Design review of the part built by this model. Coordinates are the model's own, in mm. Face numbers are marked on the shaded views. A direction names the side the tool comes from. Coordinates: 2 decimals unless noted, no trailing zeros. Loops run counter-clockwise (first coordinate to the right, second up) from the corner with the lowest first, then second, coordinate; pieces in that order, holes last.
from build123d import *

# Parameters (mm, degrees)
F_0075_CYLINDER_SKETCH_R    = 3.25
F_0075_CYLINDER_DEPTH       = 2.5
F_0076_FILLET_R             = 0.625
F_0077_EXTRUDE_DEPTH        = 1.385
F_0077_EXTRUDE_ROTATE_ANGLE = 120
F_0080_CYLINDER_SKETCH_R    = 1.2
F_0080_CYLINDER_DEPTH       = 17.7
F_0081_CONE_ROTATE_ANGLE    = 90


with BuildPart() as part:
    # 0075_cylinder_Sketch → 0075_cylinder (new body)
    with BuildSketch(Plane.XY):
        Circle(F_0075_CYLINDER_SKETCH_R)
    extrude(amount=F_0075_CYLINDER_DEPTH)

    # 0076_fillet
    f_0076_fillet_edges = [part.edges().sort_by_distance(p)[0] for p in [
        (-3.25, 0, 2.5),
    ]]
    fillet(f_0076_fillet_edges, radius=F_0076_FILLET_R)


with BuildPart() as body_2:
    # 0077_extrude_Sketch → 0077_extrude (new body)
    with BuildSketch(Plane.XY):
        Polygon((0, 0), (1.154700538, 0), (1.732050808, 1), (1.154700538, 2), (0, 2), (-0.577350269, 1), align=None)
    extrude(amount=F_0077_EXTRUDE_DEPTH)


with BuildPart() as body_2_1:
    # 0077_extrude_Rotate: read off the stored shape, not the designer's step
    # 0077_extrude_Rotate: moved
    add(body_2.part.rotate(Axis((0, 0, 0), (0, 0, 1)), F_0077_EXTRUDE_ROTATE_ANGLE))


with BuildPart() as body_2_2:
    # 0077_extrude_Translate: moved
    add(body_2_1.part.moved(Location((1.154700538, 0, 1.125))))


with BuildPart() as part_1:
    add(part.part)

    # 0079_sub: cut body 2
    add(body_2_2.part, mode=Mode.SUBTRACT)


with BuildPart() as body_2_2_1:
    # 0080_cylinder_Sketch → 0080_cylinder (new body)
    with BuildSketch(Plane.XY):
        Circle(F_0080_CYLINDER_SKETCH_R)
    extrude(amount=F_0080_CYLINDER_DEPTH)


with BuildPart() as body_2_2_2:
    # 0080_cylinder_Translate: moved
    add(body_2_2_1.part.moved(Location((0, 0, -17.7))))


with BuildPart() as body_3:
    # 0081_cone_Sketch → 0081_cone (revolve)
    with BuildSketch(Plane.XY, mode=Mode.PRIVATE) as f_0081_cone_sk:
        Polygon((0, 0), (1.2, 0), (0.9, 0.3), (0, 0.3), align=None)
    revolve(f_0081_cone_sk.sketch.rotate(Axis((0, -100, 0), (0, 1, 0)), 90), axis=Axis((0, -100, 0), (0, 1, 0)))


with BuildPart() as body_3_1:
    # 0081_cone_Rotate: moved
    add(body_3.part.rotate(Axis((0, 0, 0), (1, 0, 0)), F_0081_CONE_ROTATE_ANGLE))


with BuildPart() as body_3_2:
    # 0081_cone_Translate: moved
    add(body_3_1.part.moved(Location((0, 0, -18))))


with BuildPart() as body_2_2_3:
    add(body_2_2_2.part)

    # 0083_add: union body 3
    add(body_3_2.part)


with BuildPart() as part_2:
    add(part_1.part)

    # 0084_add: union body 2 2
    add(body_2_2_3.part)


solid = part_2.part
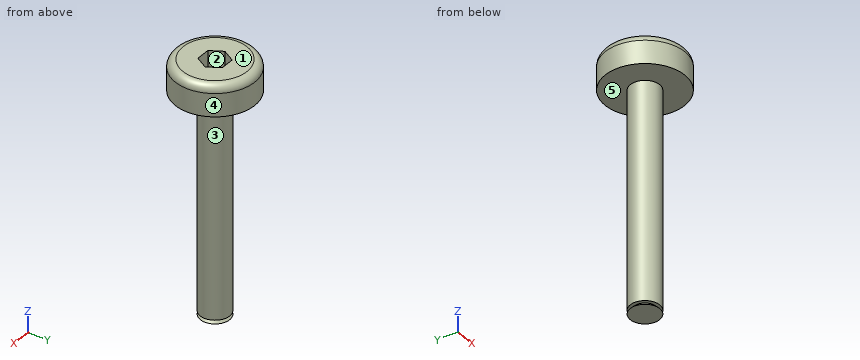
Q1. Machinability: for the marked faces 4 and 5, which of the approach directions +Z, -Z, +X, -X, +Y, -Y give a long, thin tool a straight path to every point of the face, cutting with its end or side? Answer none if there is none.
Q2. For line 1 (Z direction, x = 1, y = 1.25); line 2 (Y direction, x = 0.5, z = -13), list the stretches that pass through material, from the lowest coordinate up.
Q3. The part is to be moulded in two halves that separate along X. For the marked faces 1, 2 and 3, say which applies: pulls with the +X half, pulls with the -X half, needs draft (parallel to the pull), parting line crosses it, or undercut.
Q4. Take a section at A-A, the plane x = 0. Write out the cut boundary in (y, z) (3 decimals), then the cut area to 3 significant figures.
Q5. Clearance check with flat-ended pins moving along their axes: pin 1 Ø1.5 at (x, y) = (-2, 2) entering from +Z; pin 2 Ø2 at (y, z) = (-2, -15.5) entering from +X. State where each tip first meets the part, or that it passes through.
Q6. Take a section at C-C, the plane z = -10.25. Write out the cut boundary in (x, y).
Q7. Take a section at B-B, the plane z = 0.75. Write out the cut boundary in (x, y).
Entries:
1. face 4: +Z, -Z
1. face 5: -Z
2. line 1: z = 0 to 2.5
2. line 2: y = -1.09 to 1.09
3. face 1: needs draft
3. face 2: undercut
3. face 3: parting line crosses it
4. outline: (-3.25, 0) - (-1.2, 0) - (-1.2, -17.7) - (-0.9, -17.7) - (-1.2, -18) - (1.2, -18) - (0.9, -17.7) - (1.2, -17.7) - (1.2, 0) - (3.25, 0) - (3.25, 1.875) arc R0.625 ccw to (2.625, 2.5) - (1, 2.5) - (1, 1.125) - (-1, 1.125) - (-1, 2.5) - (-2.625, 2.5) arc R0.625 ccw to (-3.25, 1.875) - close
4. area: 56.4 mm2
5. pin 1: stops at z = 2.5
5. pin 2: stops at x = 0.66
6. outline: circle Ø2.4 at (0, 0)
7. outline: circle Ø6.5 at (0, 0)
